Check sheet for the modelled part. Datum: model origin and axes. Units: mm. Face numbers are marked on the shaded views. Round coordinates to 2 decimals unless told otherwise and drop trailing zeros. Write each loop counter-clockwise with the first axis right and the second up, starting at its lowest first coordinate (ties: lowest second). Pieces come first, ordered by that corner, then holes.
Item 1: Material ranges on line 1 (Y direction, x = -2, z = 8); line 2 (Z direction, x = 0, y = 1.3); line 3 (X direction, y = 0, z = 8.5), recorded low to high.
Item 2: Release check for a two-part mould opening along Z. For the marked faces 1, 2 and 3 record: +Z half, -Z half, draft (parallel to the pull), parting line (faces both ways), or undercut.
Item 3: Cross-section at B-B on z = 10. Enter the section's corners in (x, y).
Item 4: Cross-section at C-C on y = 0. Enter the section's corners in (x, z).
Item 5: Go/stop test with a flat-tipped pin: pin 1 Ø1 at (y, z) = (1.5, 17) entering from -X. Record where the tip stops, or that it passes through.
Item 6: Cross-section at A-A on x = 2.75. Enter the section's corners in (y, z), plus the area to 3 significant figures.
Item 7: Cross-section at D-D on z = 2. Enter the section's corners in (x, y).
from build123d import *

# Parameters (mm, degrees)
F1_DEPTH = 20
F3_R     = 2.5
F4_DEPTH = 7.001


with BuildPart() as f1:
    # F0 (on Top) → F1 (new body)
    with BuildSketch(Plane.XY):
        with BuildLine():
            ThreePointArc((3.450807, 0.7), (6.699989, 0.006025), (3.455807, -0.710963))
            Line((3.455807, -0.710963), (0, -0.710963))
            Line((0, -0.710963), (0, -3.5))
            Line((0, -3.5), (5, -3.5))
            ThreePointArc((5, -3.5), (8.5, 0), (5, 3.5))
            Line((5, 3.5), (0, 3.5))
            Line((0, 3.5), (0, 0.7))
            Line((0, 0.7), (3.450807, 0.7))
        make_face()
    extrude(amount=F1_DEPTH)

    # F2: F1 across plane


with BuildPart() as f1_1:
    add(f1.part)
    add(f1.part.mirror(Plane.YZ))

    # F3 (on face) → F4 (cut, through all)
    with BuildSketch(Plane(origin=(0, 3.5, 0), x_dir=(-1, 0, 0), z_dir=(0, 1, 0))):
        with Locations((0, 10)):
            Circle(F3_R)
    extrude(amount=-F4_DEPTH, mode=Mode.SUBTRACT)


solid = f1_1.part
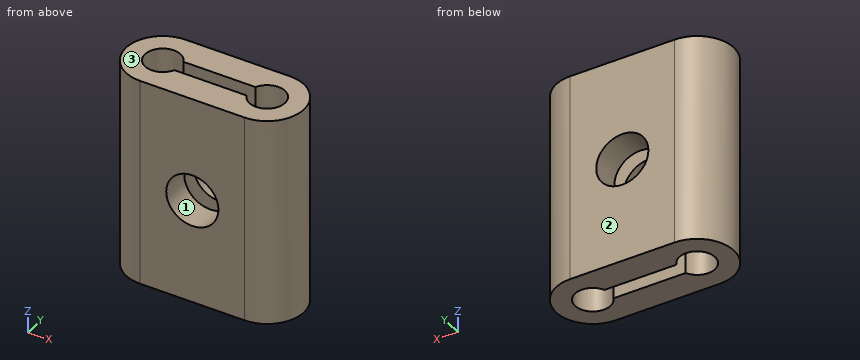
Response values:
1. line 1: y = -3.5 to -0.71, 0.7 to 3.5
1. line 2: z = 0 to 7.5, 12.5 to 20
1. line 3: x = -8.5 to -6.7, 6.7 to 8.5
2. face 1: undercut
2. face 2: draft
2. face 3: +Z half
3. outline: (-5, -3.5) - (-2.5, -3.5) - (-2.5, -0.71) - (-3.46, -0.71) arc R1.7 cw (long way) to (-3.45, 0.7) - (-2.5, 0.7) - (-2.5, 3.5) - (-5, 3.5) arc R3.5 ccw to start; (2.5, -3.5) - (5, -3.5) arc R3.5 ccw to (5, 3.5) - (2.5, 3.5) - (2.5, 0.7) - (3.45, 0.7) arc R1.7 cw (long way) to (3.46, -0.71) - (2.5, -0.71) - close
4. outline: (-8.5, 0) - (-6.7, 0) - (-6.7, 20) - (-8.5, 20) - close; (6.7, 0) - (8.5, 0) - (8.5, 20) - (6.7, 20) - close
5. pin 1: stops at x = -8.35
6. outline: (-3.5, 0) - (-0.71, 0) - (-0.71, 20) - (-3.5, 20) - close; (0.7, 0) - (3.5, 0) - (3.5, 20) - (0.7, 20) - close
6. area: 112 mm2
7. outline: (-5, -3.5) - (5, -3.5) arc R3.5 ccw to (5, 3.5) - (-5, 3.5) arc R3.5 ccw to start; hole (-3.46, -0.71) - (3.46, -0.71) arc R1.7 ccw (long way) to (3.45, 0.7) - (-3.45, 0.7) arc R1.7 ccw (long way) to start
